Geometry: see drawing. Coordinates: mm, zero at the bounding-box minimum. A direction names the side the tool comes from. Give positions to 0.01 mm unless a question says otherwise; leave off trailing zeros. Write each loop counter-clockwise with the first axis right and the second up, starting at its lowest first coordinate (ties: lowest second). Pieces come first, ordered by that corner, then holes. Notation, with made-up numbers: (-34.75, -40) - (16.25, -40) arc R31 ccw to (16.25, -2) - close; hole circle Ø9 at (13, 54.25). An arc over 180 degrees is marked (long way). Use a Markdown table: item, result. Add a question column.
1. Pin query (flat end, axial travel): pin 1 (8 mm diameter, centred on y = 12, z = 13, fed in from +X); pin 2 (5 mm diameter, centred on x = 11, y = 11, fed in from -Z); pin 3 (8 mm diameter, centred on x = 19.5, z = 12.5, fed in from -Y). Return the tip coordinate at first contact, or that it passes through.
2. Section query C-C, the plane z = 9.5. Return loops of the section in (x, y).
3. Material intervals for probe 1 along Y at (x, z) = (11, 1.15); probe 2 along Z at (x, y) = (9, 12.25); probe 3 along Z at (x, y) = (4.75, 4.5), sorted ascending.
4. Set-up query: the marked faces 1, 2 and 3. Return all of +Z, -Z, +X, -X, +Y, -Y with unobstructed straight access to the full face (end or side cutting, diameter ignored); none if empty.
5. Mould query, pull axis X, two halves, no side actions, for the marked faces 4, 5 and 6. Classes: released by +X, released by -X, zero draft, split by the parting line, or undercut.
6. Section query D-D, the plane y = 4. Return loops of the section in (x, z).
7. Section query A-A, the plane x = 11. Return loops of the section in (y, z).
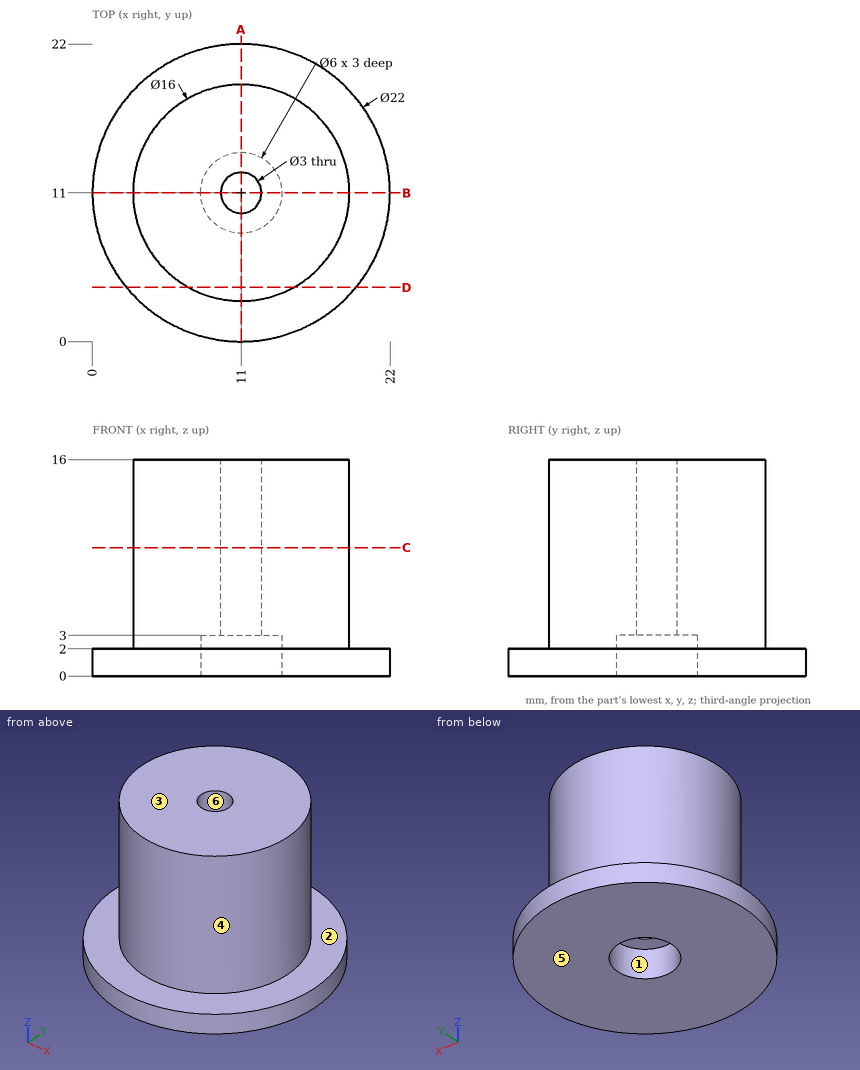
Result sheet:
| question | item | result |
|---|---|---|
| 1 | pin 1 | stops at x = 19 |
| 1 | pin 2 | stops at z = 3 |
| 1 | pin 3 | stops at y = 4.39 |
| 2 | outline | circle Ø16 at (11, 11); hole circle Ø3 at (11, 11) |
| 3 | probe 1 | y = 0 to 8, 14 to 22 |
| 3 | probe 2 | z = 3 to 16 |
| 3 | probe 3 | z = 0 to 2 |
| 4 | face 1 | -Z |
| 4 | face 2 | +Z |
| 4 | face 3 | +Z, +X, -X, +Y, -Y |
| 5 | face 4 | split by the parting line |
| 5 | face 5 | zero draft |
| 5 | face 6 | undercut |
| 6 | outline | (2.51, 0) - (19.49, 0) - (19.49, 2) - (14.87, 2) - (14.87, 16) - (7.13, 16) - (7.13, 2) - (2.51, 2) - close |
| 7 | outline | (0, 0) - (8, 0) - (8, 3) - (9.5, 3) - (9.5, 16) - (3, 16) - (3, 2) - (0, 2) - close; (12.5, 3) - (14, 3) - (14, 0) - (22, 0) - (22, 2) - (19, 2) - (19, 16) - (12.5, 16) - close |
